```python
from build123d import *

# Parameters (mm, degrees)
SKETCH_1_W          = 28
SKETCH_1_H          = 8
SKETCH_1_R          = 1.525
EXTRUDE_1_DEPTH     = 1
FILLET_1_R          = 2
SKETCH_3_R          = 1.525
CUT_EXTRUDE_1_DEPTH = 10
CUT_EXTRUDE_2_DEPTH = 10
SKETCH_5_R          = 1.525
CUT_EXTRUDE_3_DEPTH = 10
FILLET_3_R          = 2
SKETCH_8_R          = 1.525
CUT_EXTRUDE_5_DEPTH = 5
SKETCH_9_W          = 29
SKETCH_9_H          = 22
CUT_EXTRUDE_6_DEPTH = 11
FILLET_4_R          = 1
EXTRUDE_2_DEPTH     = 1
SKETCH_12_W         = 55
SKETCH_12_H         = 4.5
CUT_EXTRUDE_7_DEPTH = 10
FILLET_5_R          = 2
SKETCH_13_W         = 32
SKETCH_13_H         = 8
CUT_EXTRUDE_8_DEPTH = 10
SKETCH_14_W         = 28
SKETCH_14_H         = 8
SKETCH_14_R         = 1.525
EXTRUDE_3_DEPTH     = 1
FILLET_6_R          = 2


with BuildPart() as part:
    # 草图1 → 凸台-拉伸1 (new body)
    with BuildSketch(Plane.XY):
        Polygon((-4, 4), (24, 4), (67, 4), (67, 120), (-51, 120), (-51, 4), align=None)
        with Locations((10, 0)):
            Rectangle(SKETCH_1_W, SKETCH_1_H)
        with Locations((20, 0)):
            Circle(SKETCH_1_R, mode=Mode.SUBTRACT)
        Circle(SKETCH_1_R, mode=Mode.SUBTRACT)
    extrude(amount=EXTRUDE_1_DEPTH)

    # 圆角1
    fillet_1_edges = [part.edges().sort_by_distance(p)[0] for p in [
        (67, 4, 0.5),
        (24, 4, 0.5),
        (24, -4, 0.5),
        (-4, -4, 0.5),
        (-4, 4, 0.5),
        (-51, 4, 0.5),
        (-51, 120, 0.5),
        (67, 120, 0.5),
    ]]
    fillet(fillet_1_edges, radius=FILLET_1_R)

    # 草图3 → 切除-拉伸1 (cut)
    with BuildSketch(Plane.XY.offset(1)):
        with Locations((-48, 76.75)):
            Circle(SKETCH_3_R)
        with Locations((-48, 56.75)):
            Circle(SKETCH_3_R)
    extrude(amount=-CUT_EXTRUDE_1_DEPTH, mode=Mode.SUBTRACT)

    # 草图4 → 切除-拉伸2 (cut)
    with BuildSketch(Plane.XY.offset(1)):
        with BuildLine():
            Line((65, 120), (-24, 120))
            Line((-24, 120), (-24, 98))
            Line((-24, 98), (67, 98))
            Line((67, 98), (67, 118))
            ThreePointArc((67, 118), (66.414213562, 119.414213562), (65, 120))
        make_face()
    extrude(amount=-CUT_EXTRUDE_2_DEPTH, mode=Mode.SUBTRACT)

    # 草图5 → 切除-拉伸3 (cut)
    with BuildSketch(Plane.XY.offset(1)):
        with Locations((61, 34)):
            Circle(SKETCH_5_R)
        with Locations((61, 54)):
            Circle(SKETCH_5_R)
    extrude(amount=-CUT_EXTRUDE_3_DEPTH, mode=Mode.SUBTRACT)

    # 圆角3
    fillet_3_edges = [part.edges().sort_by_distance(p)[0] for p in [
        (-24, 98, 0.5),
        (67, 98, 0.5),
        (-24, 120, 0.5),
    ]]
    fillet(fillet_3_edges, radius=FILLET_3_R)

    # 草图8 → 切除-拉伸5 (cut, symmetric)
    with BuildSketch(Plane.XY.offset(1)):
        with Locations((12, 95)):
            Circle(SKETCH_8_R)
        with Locations((32, 95)):
            Circle(SKETCH_8_R)
    extrude(amount=CUT_EXTRUDE_5_DEPTH, both=True, mode=Mode.SUBTRACT)

    # 草图9 → 切除-拉伸6 (cut, symmetric)
    with BuildSketch(Plane.XY.offset(1)):
        with Locations((-36.5, 109)):
            Rectangle(SKETCH_9_W, SKETCH_9_H)
    extrude(amount=CUT_EXTRUDE_6_DEPTH, both=True, mode=Mode.SUBTRACT)

    # 圆角4
    fillet_4_edges = [part.edges().sort_by_distance(p)[0] for p in [
        (-51, 98, 0.5),
    ]]
    fillet(fillet_4_edges, radius=FILLET_4_R)

    # 草图11 → 凸台-拉伸2 (add)
    with BuildSketch(Plane(origin=(0, 0, 0), x_dir=(-1, 0, 0), z_dir=(0, 0, -1))):
        with BuildLine():
            ThreePointArc((-67, 96), (-66.414213562, 97.414213562), (-65, 98))
            Line((-65, 98), (-101, 98))
            Line((-101, 98), (-126.187224089, 4))
            Line((-126.187224089, 4), (-65, 4))
            ThreePointArc((-65, 4), (-66.414213562, 4.585786438), (-67, 6))
            Line((-67, 6), (-67, 96))
        make_face()
    extrude(amount=-EXTRUDE_2_DEPTH)

    # 草图12 → 切除-拉伸7 (cut)
    with BuildSketch(Plane.XY.offset(1)):
        with Locations((98.687224089, 6.25)):
            Rectangle(SKETCH_12_W, SKETCH_12_H)
    extrude(amount=-CUT_EXTRUDE_7_DEPTH, mode=Mode.SUBTRACT)

    # 圆角5
    fillet_5_edges = [part.edges().sort_by_distance(p)[0] for p in [
        (101, 98, 0.5),
        (124.981452723, 8.5, 0.5),
        (71.187224089, 4, 0.5),
        (71.187224089, 8.5, 0.5),
    ]]
    fillet(fillet_5_edges, radius=FILLET_5_R)

    # 草图13 → 切除-拉伸8 (cut)
    with BuildSketch(Plane.XY.offset(1)):
        with Locations((10, 0)):
            Rectangle(SKETCH_13_W, SKETCH_13_H)
    extrude(amount=-CUT_EXTRUDE_8_DEPTH, mode=Mode.SUBTRACT)

    # 草图14 → 凸台-拉伸3 (add)
    with BuildSketch(Plane.XY.offset(1)):
        with Locations((-17, 0)):
            Rectangle(SKETCH_14_W, SKETCH_14_H)
        with Locations((-27, 0)):
            Circle(SKETCH_14_R, mode=Mode.SUBTRACT)
        with Locations((-7, 0)):
            Circle(SKETCH_14_R, mode=Mode.SUBTRACT)
        with Locations((38, 0)):
            Rectangle(SKETCH_14_W, SKETCH_14_H)
        with Locations((28, 0)):
            Circle(SKETCH_14_R, mode=Mode.SUBTRACT)
        with Locations((48, 0)):
            Circle(SKETCH_14_R, mode=Mode.SUBTRACT)
    extrude(amount=-EXTRUDE_3_DEPTH)

    # 圆角6
    fillet_6_edges = [part.edges().sort_by_distance(p)[0] for p in [
        (52, -4, 0.5),
        (52, 4, 0.5),
        (24, 4, 0.5),
        (24, -4, 0.5),
        (-3, -4, 0.5),
        (-3, 4, 0.5),
        (-31, 4, 0.5),
        (-31, -4, 0.5),
    ]]
    fillet(fillet_6_edges, radius=FILLET_6_R)


solid = part.part
```
For this review, take the finished solid that the model builds, in its own axes (mm). Give positions to 0.01 mm unless a question says otherwise; leave off trailing zeros. Loops run counter-clockwise (first coordinate to the right, second up) from the corner with the lowest first, then second, coordinate; pieces in that order, holes last. Notation, with made-up numbers: M -2.75,-9.75 L 43.25,-9.75 A11 ccw 43.25,-1.75 Z; hole C 13.25,11 d10. An arc over 180 degrees is marked long. One line per item, written item: value. Start each with the question number.
Q1. Add section A-A (z = 0.8). Count the separate pieces of the cut face and the enclosed holes in it, and give its area (3 significant figures).
Q2. Add section C-C (y = 62). Give the boundary of the cut face in (x, z), and give its area (3 significant figures).
Q3. Clearance check with flat-ended pins moving along their axes: pin 1 Ø0.5 at (x, z) = (15, 0.5) entering from -Y; pin 2 Ø0.5 at (x, z) = (99.5, 0.5) entering from -Y; pin 3 Ø0.5 at (y, z) = (0.5, 0.5) entering from -X; pin 4 Ø2.5 at (x, y) = (12, 95) entering from +Z. State where each tip first meets the part, or that it passes through.
Q4. For L1, parallel to Y at x = 32, z = 0.6 (3 decimals); L2, parallel to X at y = 11, z = 0.6; L3, parallel to Y at x = -27, z = 0.4 (3 decimals), list the stretches that pass through material, from the lowest coordinate up.
Q5. Add section B-B (x = 94). Give the boundary of the cut face in (y, z).
Reply:
1. separate pieces: 1
1. enclosed holes: 10
1. area: 15,600 mm²
2. outline: M -51,0 L 110.65,0 L 110.65,1 L -51,1 Z
2. area: 162 mm²
3. pin 1: y = 4
3. pin 2: y = 8.5
3. pin 3: x = -31
3. pin 4: through
4. L1: -4 to 93.475, 96.525 to 98
4. L2: -51 to 124.31
4. L3: -4 to -1.525, 1.525 to 98
5. outline: M 8.5,0 L 98,0 L 98,1 L 8.5,1 Z
